```python
from build123d import *

# Parameters (mm, degrees)
SKETCH1_R           = 50
SKETCH1_R_2         = 18
SKETCH1_R_3         = 1.75
BOSS_EXTRUDE1_DEPTH = 2


with BuildPart() as part:
    # Sketch1 → Boss-Extrude1 (new body)
    with BuildSketch(Plane.XY):
        Circle(SKETCH1_R)
        Circle(SKETCH1_R_2, mode=Mode.SUBTRACT)
        with Locations((0, 22)):
            Circle(SKETCH1_R_3, mode=Mode.SUBTRACT)
        with Locations((19.052558883, -11)):
            Circle(SKETCH1_R_3, mode=Mode.SUBTRACT)
        with Locations((-19.052558883, -11)):
            Circle(SKETCH1_R_3, mode=Mode.SUBTRACT)
        with BuildLine():
            Line((25, 0), (46.5, 0))
            ThreePointArc((46.5, 0), (45.862280471, 7.674713673), (43.966613765, 15.138919182))
            Line((43.966613765, 15.138919182), (23.63796439, 8.139203861))
            ThreePointArc((23.63796439, 8.139203861), (24.657140038, 4.126190147), (25, 0))
        make_face(mode=Mode.SUBTRACT)
        with BuildLine():
            Line((23.096988313, -9.567085809), (42.960398262, -17.794779605))
            ThreePointArc((42.960398262, -17.794779605), (45.308208013, -10.460224027), (46.413268127, -2.838757088))
            Line((46.413268127, -2.838757088), (24.953369961, -1.526213488))
            ThreePointArc((24.953369961, -1.526213488), (24.35925162, -5.623776359), (23.096988313, -9.567085809))
        make_face(mode=Mode.SUBTRACT)
        with BuildLine():
            Line((17.67766953, -17.67766953), (32.880465325, -32.880465325))
            ThreePointArc((32.880465325, -32.880465325), (37.856371604, -27.002687441), (41.793923153, -20.384258326))
            Line((41.793923153, -20.384258326), (22.469851157, -10.95927867))
            ThreePointArc((22.469851157, -10.95927867), (20.352887959, -14.517573893), (17.67766953, -17.67766953))
        make_face(mode=Mode.SUBTRACT)
        with BuildLine():
            Line((9.567085809, -23.096988313), (17.794779605, -42.960398262))
            ThreePointArc((17.794779605, -42.960398262), (24.641245787, -39.434236471), (30.811832242, -34.826441017))
            Line((30.811832242, -34.826441017), (16.565501205, -18.72389302))
            ThreePointArc((16.565501205, -18.72389302), (13.247981606, -21.201202404), (9.567085809, -23.096988313))
        make_face(mode=Mode.SUBTRACT)
        with BuildLine():
            Line((0, -25), (0, -46.5))
            ThreePointArc((0, -46.5), (7.674713673, -45.862280471), (15.138919182, -43.966613765))
            Line((15.138919182, -43.966613765), (8.139203861, -23.63796439))
            ThreePointArc((8.139203861, -23.63796439), (4.126190147, -24.657140038), (0, -25))
        make_face(mode=Mode.SUBTRACT)
        with BuildLine():
            Line((-9.567085809, -23.096988313), (-17.794779605, -42.960398262))
            ThreePointArc((-17.794779605, -42.960398262), (-10.460224027, -45.308208013), (-2.838757088, -46.413268127))
            Line((-2.838757088, -46.413268127), (-1.526213488, -24.953369961))
            ThreePointArc((-1.526213488, -24.953369961), (-5.623776359, -24.35925162), (-9.567085809, -23.096988313))
        make_face(mode=Mode.SUBTRACT)
        with BuildLine():
            Line((-17.67766953, -17.67766953), (-32.880465325, -32.880465325))
            ThreePointArc((-32.880465325, -32.880465325), (-27.002687441, -37.856371604), (-20.384258326, -41.793923153))
            Line((-20.384258326, -41.793923153), (-10.95927867, -22.469851157))
            ThreePointArc((-10.95927867, -22.469851157), (-14.517573893, -20.352887959), (-17.67766953, -17.67766953))
        make_face(mode=Mode.SUBTRACT)
        with BuildLine():
            Line((-23.096988313, -9.567085809), (-42.960398262, -17.794779605))
            ThreePointArc((-42.960398262, -17.794779605), (-39.434236471, -24.641245787), (-34.826441017, -30.811832242))
            Line((-34.826441017, -30.811832242), (-18.72389302, -16.565501205))
            ThreePointArc((-18.72389302, -16.565501205), (-21.201202404, -13.247981606), (-23.096988313, -9.567085809))
        make_face(mode=Mode.SUBTRACT)
        with BuildLine():
            Line((-25, 0), (-46.5, 0))
            ThreePointArc((-46.5, 0), (-45.862280471, -7.674713673), (-43.966613765, -15.138919182))
            Line((-43.966613765, -15.138919182), (-23.63796439, -8.139203861))
            ThreePointArc((-23.63796439, -8.139203861), (-24.657140038, -4.126190147), (-25, 0))
        make_face(mode=Mode.SUBTRACT)
        with BuildLine():
            Line((-23.096988313, 9.567085809), (-42.960398262, 17.794779605))
            ThreePointArc((-42.960398262, 17.794779605), (-45.308208013, 10.460224027), (-46.413268127, 2.838757088))
            Line((-46.413268127, 2.838757088), (-24.953369961, 1.526213488))
            ThreePointArc((-24.953369961, 1.526213488), (-24.35925162, 5.623776359), (-23.096988313, 9.567085809))
        make_face(mode=Mode.SUBTRACT)
        with BuildLine():
            Line((-17.67766953, 17.67766953), (-32.880465325, 32.880465325))
            ThreePointArc((-32.880465325, 32.880465325), (-37.856371604, 27.002687441), (-41.793923153, 20.384258326))
            Line((-41.793923153, 20.384258326), (-22.469851157, 10.95927867))
            ThreePointArc((-22.469851157, 10.95927867), (-20.352887959, 14.517573893), (-17.67766953, 17.67766953))
        make_face(mode=Mode.SUBTRACT)
        with BuildLine():
            Line((-9.567085809, 23.096988313), (-17.794779605, 42.960398262))
            ThreePointArc((-17.794779605, 42.960398262), (-24.641245787, 39.434236471), (-30.811832242, 34.826441017))
            Line((-30.811832242, 34.826441017), (-16.565501205, 18.72389302))
            ThreePointArc((-16.565501205, 18.72389302), (-13.247981606, 21.201202404), (-9.567085809, 23.096988313))
        make_face(mode=Mode.SUBTRACT)
        with BuildLine():
            Line((0, 25), (0, 46.5))
            ThreePointArc((0, 46.5), (-7.674713673, 45.862280471), (-15.138919182, 43.966613765))
            Line((-15.138919182, 43.966613765), (-8.139203861, 23.63796439))
            ThreePointArc((-8.139203861, 23.63796439), (-4.126190147, 24.657140038), (0, 25))
        make_face(mode=Mode.SUBTRACT)
        with BuildLine():
            Line((9.567085809, 23.096988313), (17.794779605, 42.960398262))
            ThreePointArc((17.794779605, 42.960398262), (10.460224027, 45.308208013), (2.838757088, 46.413268127))
            Line((2.838757088, 46.413268127), (1.526213488, 24.953369961))
            ThreePointArc((1.526213488, 24.953369961), (5.623776359, 24.35925162), (9.567085809, 23.096988313))
        make_face(mode=Mode.SUBTRACT)
        with BuildLine():
            Line((17.67766953, 17.67766953), (32.880465325, 32.880465325))
            ThreePointArc((32.880465325, 32.880465325), (27.002687441, 37.856371604), (20.384258326, 41.793923153))
            Line((20.384258326, 41.793923153), (10.95927867, 22.469851157))
            ThreePointArc((10.95927867, 22.469851157), (14.517573893, 20.352887959), (17.67766953, 17.67766953))
        make_face(mode=Mode.SUBTRACT)
        with BuildLine():
            Line((23.096988313, 9.567085809), (42.960398262, 17.794779605))
            ThreePointArc((42.960398262, 17.794779605), (39.434236471, 24.641245787), (34.826441017, 30.811832242))
            Line((34.826441017, 30.811832242), (18.72389302, 16.565501205))
            ThreePointArc((18.72389302, 16.565501205), (21.201202404, 13.247981606), (23.096988313, 9.567085809))
        make_face(mode=Mode.SUBTRACT)
    extrude(amount=BOSS_EXTRUDE1_DEPTH)


solid = part.part
```
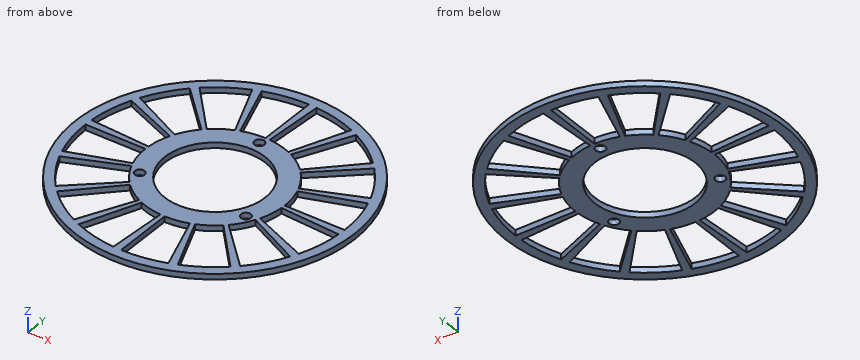
Verification items for the finished model (mm, model axes). Coordinates: 2 decimals unless noted, no trailing zeros. Loops run counter-clockwise (first coordinate to the right, second up) from the corner with the lowest first, then second, coordinate; pieces in that order, holes last. Notation, with made-up numbers: (-21.75, 2.25) -> (17.25, 2.25) arc R27 cw to (17.25, 31.25) -> close; hole circle Ø11 at (29, 31). An arc over 180 degrees is marked (long way). Answer in a Markdown table with one row per item.
1) Section check C-C (z = 1.45). Give the number of separate pieces and of enclosed holes in the cut face, and give its area (3 significant figures).
The answers:
| item | result |
|---|---|
| separate pieces | 1 |
| enclosed holes | 20 |
| area | 2,730 mm2 |
2) Depth check by flat-ended pin: P1, Ø1, axis at x = 12, z = 1.5, coming from the +Y side; P2, Ø0.6, axis at y = -34.5, z = 0.5, coming from the +X side; P3, Ø0.6, axis at x = 39.5, z = 1, coming from the +Y side. Enter the tip coordinate at first touch or a pass-through.
The answers:
| item | result |
|---|---|
| P1 | stops at y = 48.66 |
| P2 | stops at x = 36.47 |
| P3 | stops at y = 31.04 |
3) Section check A-A (x = -27). Record the cut outline in (y, z).
The answers:
| item | result |
|---|---|
| outline | (-42.08, 0) -> (-37.86, 0) -> (-37.86, 2) -> (-42.08, 2) -> close; (-27, 0) -> (-23.89, 0) -> (-23.89, 2) -> (-27, 2) -> close; (-11.18, 0) -> (-9.3, 0) -> (-9.3, 2) -> (-11.18, 2) -> close; (0, 0) -> (1.65, 0) -> (1.65, 2) -> (0, 2) -> close; (11.18, 0) -> (13.17, 0) -> (13.17, 2) -> (11.18, 2) -> close; (27, 0) -> (30.52, 0) -> (30.52, 2) -> (27, 2) -> close; (37.86, 0) -> (42.08, 0) -> (42.08, 2) -> (37.86, 2) -> close |
4) Scan lines: line 1 along X through (y, z) = (0.5, 1) (1 decimal); line 2 along Y through (x, z) = (-20, 0.45); line 3 along Y through (x, z) = (42, 0.9). Record each from-to range of solid material in increasing order. Write a range as from..to.
The answers:
| item | result |
|---|---|
| line 1 | x = -50..-18, 18..25, 46.5..50 |
| line 2 | y = -45.83..-41.01, -20..-17.69, -15..-12.47, -9.53..15, 20..22.61, 41.98..45.83 |
| line 3 | y = -27.13..-17.4, -2.57..0, 14.46..17.4, 19.96..27.13 |
5) Section check B-B (y = -27). Record the cut outline in (x, z).
The answers:
| item | result |
|---|---|
| outline | (-42.08, 0) -> (-37.86, 0) -> (-37.86, 2) -> (-42.08, 2) -> close; (-30.52, 0) -> (-27, 0) -> (-27, 2) -> (-30.52, 2) -> close; (-13.17, 0) -> (-11.18, 0) -> (-11.18, 2) -> (-13.17, 2) -> close; (-1.65, 0) -> (0, 0) -> (0, 2) -> (-1.65, 2) -> close; (9.3, 0) -> (11.18, 0) -> (11.18, 2) -> (9.3, 2) -> close; (23.89, 0) -> (27, 0) -> (27, 2) -> (23.89, 2) -> close; (37.86, 0) -> (42.08, 0) -> (42.08, 2) -> (37.86, 2) -> close |
